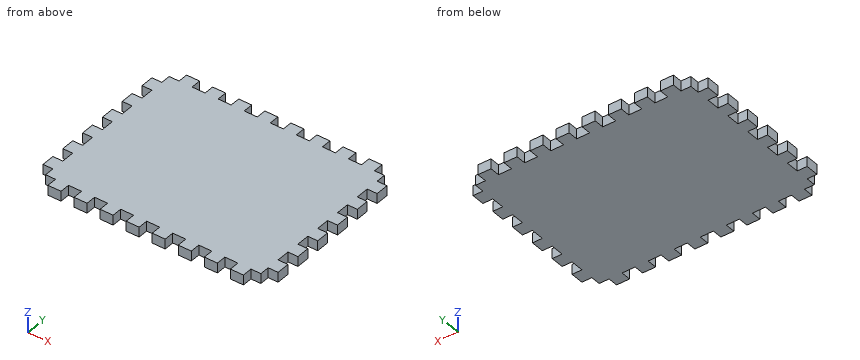
from build123d import *

# Parameters (mm, degrees)
F1_DEPTH = 9.652


with BuildPart() as f1:
    # F0 (on Top) → F1 (new body)
    with BuildSketch(Plane.XY):
        Polygon((32.004, 0), (19.304, 0), (19.304, -9.652), (9.652, -9.652), (9.652, -19.05), (0, -19.05), (0, -31.75), (9.652, -31.75), (9.652, -44.45), (0, -44.45), (0, -57.15), (9.652, -57.15), (9.652, -69.85), (0, -69.85), (0, -82.55), (9.652, -82.55), (9.652, -95.25), (0, -95.25), (0, -107.95), (9.652, -107.95), (9.652, -120.65), (0, -120.65), (0, -133.35), (9.652, -133.35), (9.652, -146.05), (0, -146.05), (0, -158.75), (9.652, -158.75), (9.652, -168.148), (19.304, -168.148), (19.304, -177.8), (32.004, -177.8), (32.004, -168.148), (44.704, -168.148), (44.704, -177.8), (57.404, -177.8), (57.404, -168.148), (70.104, -168.148), (70.104, -177.8), (82.804, -177.8), (82.804, -168.148), (95.504, -168.148), (95.504, -177.8), (108.204, -177.8), (108.204, -168.148), (120.904, -168.148), (120.904, -177.8), (133.604, -177.8), (133.604, -168.148), (146.304, -168.148), (146.304, -177.8), (159.004, -177.8), (159.004, -168.148), (171.704, -168.148), (171.704, -177.8), (184.404, -177.8), (184.404, -168.148), (197.104, -168.148), (197.104, -177.8), (209.804, -177.8), (209.804, -168.148), (219.456, -168.148), (219.456, -158.75), (229.108, -158.75), (229.108, -146.05), (219.456, -146.05), (219.456, -133.35), (229.108, -133.35), (229.108, -120.65), (219.456, -120.65), (219.456, -107.95), (229.108, -107.95), (229.108, -95.25), (219.456, -95.25), (219.456, -82.55), (229.108, -82.55), (229.108, -69.85), (219.456, -69.85), (219.456, -57.15), (229.108, -57.15), (229.108, -44.45), (219.456, -44.45), (219.456, -31.75), (229.108, -31.75), (229.108, -19.05), (219.456, -19.05), (219.456, -9.652), (209.804, -9.652), (209.804, 0), (197.104, 0), (197.104, -9.652), (184.404, -9.652), (184.404, 0), (171.704, 0), (171.704, -9.652), (159.004, -9.652), (159.004, 0), (146.304, 0), (146.304, -9.652), (133.604, -9.652), (133.604, 0), (120.904, 0), (120.904, -9.652), (108.204, -9.652), (108.204, 0), (95.504, 0), (95.504, -9.652), (82.804, -9.652), (82.804, 0), (70.104, 0), (70.104, -9.652), (57.404, -9.652), (57.404, 0), (44.704, 0), (44.704, -9.652), (32.004, -9.652), align=None)
    extrude(amount=F1_DEPTH)


solid = f1.part
Geometry: final body of the model. Coordinates: model frame, mm. Coordinates: 2 decimals unless noted, no trailing zeros. Loops run counter-clockwise (first coordinate to the right, second up) from the corner with the lowest first, then second, coordinate; pieces in that order, holes last. Notation, with made-up numbers: (-39.5, 26.25) - (-13.5, 26.25) arc R15 cw to (-13.5, 37.25) - close; hole circle Ø5 at (62, 44.25). An arc over 180 degrees is marked (long way). Put each result on its own line as item: value. Start each with the question number.
Q1. Line query: line 1 (Y direction, x = 213, z = 3.25); line 2 (X direction, y = -60, z = 4). Output: solid intervals per line, ascending.
Q2. Cut plane B-B, the plane x = 142. Return loops of the section in (y, z).
Q3. Cut plane A-A, the plane y = -118. Return loops of the section in (x, z).
Q4. Pin query (flat end, axial travel): pin 1 Ø3 at (y, z) = (-5.5, 6) entering from +X; pin 2 Ø2 at (y, z) = (-62, 6) entering from +X; pin 3 Ø5 at (y, z) = (-172.5, 3) entering from -X; pin 4 Ø1.5 at (x, z) = (31, 6.5) entering from +Y. Return the tip coordinate at first contact, or that it passes through.
Filled sheet:
1. line 1: -168.15 to -9.65
1. line 2: 9.65 to 219.46
2. outline: (-168.15, 0) - (-9.65, 0) - (-9.65, 9.65) - (-168.15, 9.65) - close
3. outline: (9.65, 0) - (219.46, 0) - (219.46, 9.65) - (9.65, 9.65) - close
4. pin 1: x = 209.8
4. pin 2: x = 219.46
4. pin 3: x = 19.3
4. pin 4: y = 0
